Could you check a few things on this model? Use its own coordinates, in mm. A direction names the side the tool comes from. Coordinates: 2 decimals unless noted, no trailing zeros. Loops run counter-clockwise (first coordinate to the right, second up) from the corner with the lowest first, then second, coordinate; pieces in that order, holes last.
from build123d import *

# Parameters (mm, degrees)
BOSS_EXTRUDE1_DEPTH = 60
SKETCH2_R           = 2
BOSS_EXTRUDE2_DEPTH = 50


with BuildPart() as part:
    # Sketch1 → Boss-Extrude1 (new body, symmetric)
    with BuildSketch(Plane(origin=(0, 0, 0), x_dir=(0, 0, -1), z_dir=(1, 0, 0))):
        with BuildLine():
            Line((-1.322875656, 1.5), (1.322875656, 1.5))
            ThreePointArc((1.322875656, 1.5), (0, -2), (-1.322875656, 1.5))
        make_face()
    extrude(amount=BOSS_EXTRUDE1_DEPTH, both=True)

    # Sketch2 → Boss-Extrude2 (add, symmetric)
    with BuildSketch(Plane(origin=(0, 0, 0), x_dir=(0, 0, -1), z_dir=(1, 0, 0))):
        Circle(SKETCH2_R)
    extrude(amount=BOSS_EXTRUDE2_DEPTH, both=True)


solid = part.part
1) Imagine slicing it at B-B on x = 16. List the corners of the cut face in (y, z) for me.
2) Imagine slicing it at C-C on y = -0.95. List the corners of the cut face in (x, z) for me, plus the area to 3 significant figures.
3) For faces 1 (the flat face through (55, 1.5, 0)), 2 (the flat face through (60, 0, 0)), 3 (the flat face through (-55, 1.5, 0)), which set-ups out of +Z, -Z, +X, -X, +Y, -Y let a thin tool reach every point of the face, with its end or its side?
4) If I drill on L1, parallel to Z at x = 6, y = 0.15; L2, parallel to Y at x = 51.5, z = 1.5; L3, parallel to X at y = 1.6, z = -0.5, over which ranges is the centre line in solid material (lowest first)?
5) Will this pin go through, and if not, where does the flat tip stop? pin 1 (1.3 mm diameter, centred on x = -54.5, z = -0.5, fed in from +Y).
6) Imagine slicing it at A-A on z = 0. List the corners of the cut face in (x, y) for me, plus the area to 3 significant figures.
Solved:
1. outline: circle Ø4 at (0, 0)
2. outline: (-60, -1.76) - (60, -1.76) - (60, 1.76) - (-60, 1.76) - close
2. area: 422 mm2
3. face 1: +Z, -Z, +X, +Y
3. face 2: +Z, -Z, +X, +Y, -Y
3. face 3: +Z, -Z, -X, +Y
4. L1: z = -1.99 to 1.99
4. L2: y = -1.32 to 1.32
4. L3: x = -50 to 50
5. pin 1: stops at y = 1.5
6. outline: (-60, -2) - (60, -2) - (60, 1.5) - (50, 1.5) - (50, 2) - (-50, 2) - (-50, 1.5) - (-60, 1.5) - close
6. area: 470 mm2
